Design review of the part shown in the three views and the two pictorial views. Dimensions are in mm from the part's minimum x, y and z. A direction names the side the tool comes from. Round coordinates to 2 decimals unless told otherwise and drop trailing zeros. Order: outer loops, then holes, each group sorted by start corner. A loop starts at its lowest first (then second) coordinate and runs counter-clockwise, first axis right, second up. Notation, with made-up numbers: (71, 16) - (107, 16) arc R26 cw to (107, 51) - close; hole circle Ø3 at (23, -12.5). An arc over 180 degrees is marked (long way). One line per question, with ' | ' between items. Start each with the question number.
Item 1: Add section C-C on x = 5. State the section outline as (y, z) points.
Item 2: Add section B-B on y = 5. State the section outline as (x, z) points, and give its area (3 significant figures).
Item 3: For L1, parallel to X at y = 6.5, z = 2.5; L2, parallel to Z at x = 5.5, y = 7; L3, parallel to Y at x = 5.5, z = 8.5 (1 decimal), list the stretches that pass through material, from the lowest coordinate up. Write a range as [from, to].
Item 4: Insertion check: pin 1 Ø5 at (y, z) = (1.5, 5) entering from -X; pin 2 Ø4 at (x, z) = (8.5, 7.5) entering from +Y; pin 3 Ø3 at (x, y) = (5, 5) entering from -Z. Each pin has a flat end and moves straight along its axis. Give the tip position at first contact, or say it passes through.
Item 5: Draft analysis for pull direction Y (two halves, no side actions). For the marked faces 1, 2 and 3, state which applies: +Y half, -Y half, draft (parallel to the pull), parting line (faces both ways), or undercut.
Item 6: Tool access review of the marked faces 4, 5 and 6: name each direction out of +Z, -Z, +X, -X, +Y, -Y from which nothing blocks a thin tool from reaching the whole face with its end or side.
Item 7: Add section A-A on z = 5. State the section outline as (x, y) points (1 decimal).
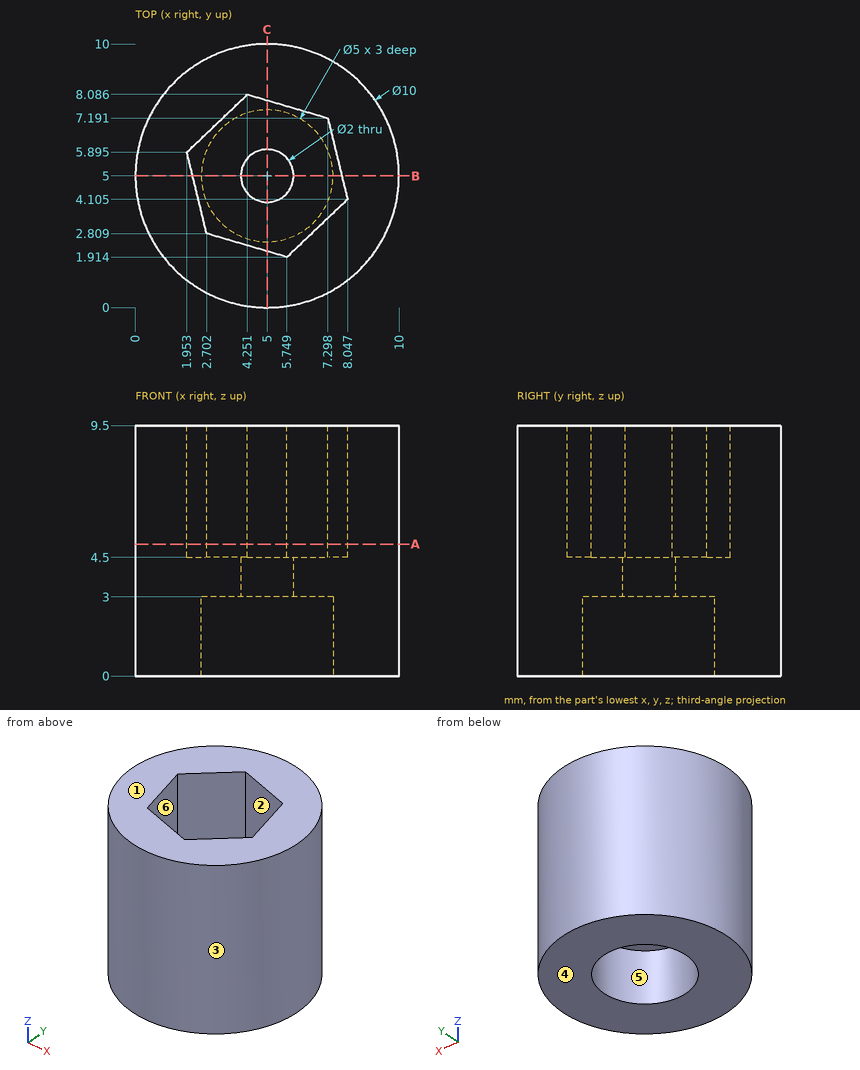
Determined:
1) outline: (0, 0) - (2.5, 0) - (2.5, 3) - (4, 3) - (4, 4.5) - (2.13, 4.5) - (2.13, 9.5) - (0, 9.5) - close; (6, 3) - (7.5, 3) - (7.5, 0) - (10, 0) - (10, 9.5) - (7.87, 9.5) - (7.87, 4.5) - (6, 4.5) - close
2) outline: (0, 0) - (2.5, 0) - (2.5, 3) - (4, 3) - (4, 4.5) - (2.17, 4.5) - (2.17, 9.5) - (0, 9.5) - close; (6, 3) - (7.5, 3) - (7.5, 0) - (10, 0) - (10, 9.5) - (7.83, 9.5) - (7.83, 4.5) - (6, 4.5) - close | area: 48.7 mm2
3) L1: [0.23, 3], [7, 9.77] | L2: [3, 4.5] | L3: [0, 2], [7.7, 10]
4) pin 1: x = 0.1 | pin 2: y = 9.77 | pin 3: z = 3
5) face 1: draft | face 2: undercut | face 3: parting line
6) face 4: -Z, +X, -X, +Y, -Y | face 5: -Z | face 6: +Z
7) outline: circle Ø10 at (5, 5); hole (2, 5.9) - (2.7, 2.8) - (5.7, 1.9) - (8, 4.1) - (7.3, 7.2) - (4.3, 8.1) - close
